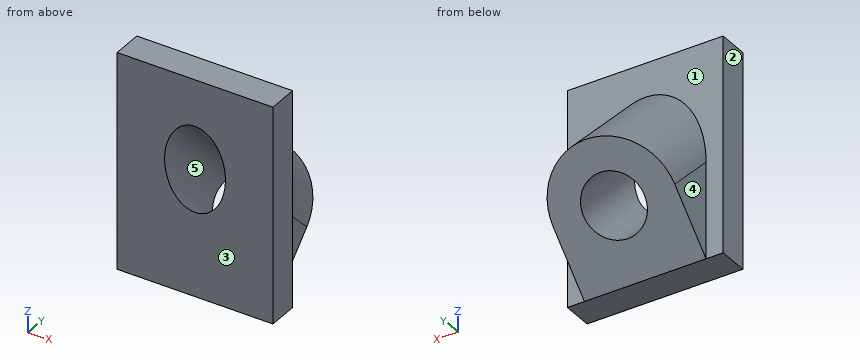
```python
from build123d import *

# Parameters (mm, degrees)
SKETCH_1_W          = 57
SKETCH_1_H          = 8
EXTRUDE_1_DEPTH     = 41
EXTRUDE_2_REACH     = 65.274
SKETCH_3_R          = 8
CUT_EXTRUDE_1_DEPTH = 41


with BuildPart() as part:
    # 草图1 → 凸台-拉伸1 (new body)
    with BuildSketch(Plane(origin=(0, 0, 0), x_dir=(0, 0, -1), z_dir=(1, 0, 0))):
        with Locations((0, -4)):
            Rectangle(SKETCH_1_W, SKETCH_1_H)
    extrude(amount=-EXTRUDE_1_DEPTH)

    # 草图2 → 凸台-拉伸2 (add, up to next)
    with BuildSketch(Plane(origin=(0, 14.25, -14.25), x_dir=(1, 0, 0), z_dir=(0, 0.7071067811865488, -0.7071067811865464)), mode=Mode.PRIVATE) as extrude_2_sk1:
        with BuildLine():
            Line((-36.5, 2.152543264), (-36.5, 20.152543264))
            Line((-36.5, 20.152543264), (-4.5, 20.152543264))
            Line((-4.5, 20.152543264), (-4.5, 2.152543264))
            ThreePointArc((-4.5, 2.152543264), (-20.5, -13.847456736), (-36.5, 2.152543264))
        make_face()
    extrude_2_tool1 = extrude(extrude_2_sk1.sketch, amount=-EXTRUDE_2_REACH, mode=Mode.PRIVATE) - part.part
    add(extrude_2_tool1.solids().sort_by_distance((-20.5, 10.954355, -17.545645))[0])

    # 草图3 → 切除-拉伸1 (cut)
    with BuildSketch(Plane(origin=(0, 14.25, -14.25), x_dir=(1, 0, 0), z_dir=(0, 0.7071067811865488, -0.7071067811865464))):
        with Locations(Location((-20.5, 2.152543264, 0), (0, 0, 270))):
            Circle(SKETCH_3_R)
    extrude(amount=-CUT_EXTRUDE_1_DEPTH, mode=Mode.SUBTRACT)


solid = part.part
```
Geometry check sheet. Reference: the model listing, model coordinates, mm. Face numbers are marked on the shaded views. A direction names the side the tool comes from. Give positions to 0.01 mm unless a question says otherwise; leave off trailing zeros. Write each loop counter-clockwise with the first axis right and the second up, starting at its lowest first coordinate (ties: lowest second). Pieces come first, ordered by that corner, then holes. Notation, with made-up numbers: (-23.5, 42.25) - (12.5, 42.25) arc R20 cw to (12.5, 75.25) - close; hole circle Ø8 at (44.5, -35.5). An arc over 180 degrees is marked (long way). Use a Markdown table: item, result.
Q1. Section check C-C, the plane x = -17. Enter the section's corners in (y, z), then the cut area to 3 significant figures.
Computed:
| item | result |
|---|---|
| outline | (-8, -28.5) - (0, -28.5) - (7.64, -20.86) - (-8, -5.22) - close; (-8, 15.13) - (17.81, -10.69) - (23.77, -4.73) - (0, 19.04) - (0, 28.5) - (-8, 28.5) - close |
| area | 599 mm² |
Q2. Section check B-B, the plane z = -23.5. Enter the section's corners in (x, y), then the cut area to 3 significant figures.
Computed:
| item | result |
|---|---|
| outline | (-41, -8) - (0, -8) - (0, 0) - (-4.5, 0) - (-4.5, 5) - (-36.5, 5) - (-36.5, 0) - (-41, 0) - close |
| area | 488 mm² |
Q3. Draft check along X on the marked faces 3, 4 and 5. Enter one of: pulls with the +X half, pulls with the -X half, needs draft (parallel to the pull), parting line crosses it, or undercut.
Computed:
| item | result |
|---|---|
| face 3 | needs draft |
| face 4 | pulls with the -X half |
| face 5 | undercut |
Q4. Thickness scan on L1, parallel to Y at x = -37.5, z = 14.5; L2, parallel to X at y = 9, z = -17; L3, parallel to X at y = -6, z = 11.5. Record the ranges inside material, lowest first. Write a range as [from, to].
Computed:
| item | result |
|---|---|
| L1 | y = [-8, 0] |
| L2 | x = [-36.5, -27.69], [-13.31, -4.5] |
| L3 | x = [-41, -25.74], [-15.26, 0] |
Q5. Set-up check for the marked faces 1 and 2: record each of +Z, -Z, +X, -X, +Y, -Y from which the full face is reachable in a straight line by a thin tool's end or side.
Computed:
| item | result |
|---|---|
| face 1 | +Z, +Y |
| face 2 | +Z, -Z, -X, +Y, -Y |
Q6. Go/stop test with flat-tipped pins: P1, Ø12, axis at y = -4, z = -22.5, coming from the +X side; P2, Ø5, axis at x = -36, z = 15.5, coming from the +Y side; P3, Ø2, axis at x = -25.5, y = 17, coming from the +Z side; P4, Ø12.5, axis at x = -16, z = 2.5, coming from the +Y side. Record where each tip stops, or that it passes through.
Computed:
| item | result |
|---|---|
| P1 | stops at x = 0 |
| P2 | stops at y = 0 |
| P3 | stops at z = 2.54 |
| P4 | stops at y = 22.75 |
Q7. Section check A-A, the plane x = -25. Enter the section's corners in (y, z) (3 decimals), then the cut area to 3 significant figures.
Computed:
| item | result |
|---|---|
| outline | (-8, -28.5) - (0, -28.5) - (8.051, -20.449) - (-8, -4.398) - close; (-8, 14.31) - (17.405, -11.095) - (23.585, -4.915) - (0, 18.67) - (0, 28.5) - (-8, 28.5) - close |
| area | 624 mm² |
